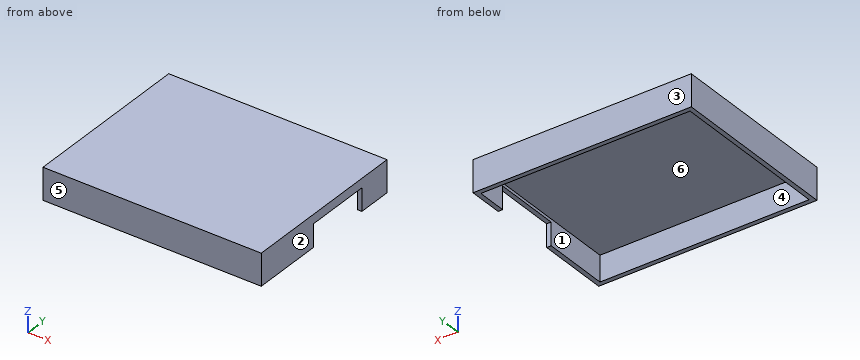
Autodesk Inventor part; units mm, degrees
ref_plane "Plan de construction1" through (-50.5759, 25.8928, -3.5) normal (-1, 0, 0) x (0, 0, 1)
ref_plane "YZ Plane" through (0, 0, 0) normal (1, 0, 0) x (0, 1, 0)
ref_plane "XZ Plane" through (0, 0, 0) normal (0, 1, 0) x (-1, 0, 0)
sketch "Esquisse1" plane through (0, 0, 0) normal (0, 0, 1) x (1, 0, 0)
  line L0 (-45.5759, 93.3928) -> (-189.5759, 93.3928)
  line L1 (-189.5759, 93.3928) -> (-189.5759, -20.6072)
  line L2 (-45.5759, -20.6072) -> (-45.5759, 93.3928)
  line L3 (-189.5759, -20.6072) -> (-45.5759, -20.6072)
  line L4 (-189.5759, 93.3928) -> (-45.5759, 93.3928)
  line L5 (-45.5759, 93.3928) -> (-45.5759, -20.6072)
  line L6 (-45.5759, -20.6072) -> (-189.5759, -20.6072)
  line L7 (-189.5759, -20.6072) -> (-189.5759, 93.3928)
  point P0 (0, 0)
extrude "Extrusion1" add sketch "Esquisse1" along normal blind 21
sketch "Esquisse2" plane through (0, 0, 0) normal (0, 0, -1) x (-1, 0, 0)
  line L0 (186.5759, -17.6072) -> (48.5759, -17.6072)
  line L1 (48.5759, -17.6072) -> (48.5759, 90.3928)
  line L2 (48.5759, 90.3928) -> (186.5759, 90.3928)
  line L3 (186.5759, 90.3928) -> (186.5759, -17.6072)
  line L4 (189.5759, -20.6072) -> (45.5759, -20.6072)
  line L5 (45.5759, 93.3928) -> (189.5759, 93.3928)
  line L6 (189.5759, 93.3928) -> (189.5759, -20.6072)
  line L7 (45.5759, -20.6072) -> (45.5759, 93.3928)
  point P0 (0, 0)
  dimension "d2" = 3
  dimension "d4" = 3
  dimension "d5" = 3
  dimension "d6" = 3
extrude "Extrusion3" cut sketch "Esquisse2" against normal blind 17 contours L0 L1 L2 L3
sketch "Esquisse3" plane through (-45.5759, -20.6072, 0) normal (1, 0, 0) x (0, 0, -1)
  line L0 (-15, 47.25) -> (0, 47.25)
  line L1 (0, 47.25) -> (0, 91.25)
  line L2 (0, 91.25) -> (-15, 91.25)
  line L3 (-15, 91.25) -> (-15, 47.25)
  line L4 (0, -22.8) -> (0, 136.8)
  line L5 (0, 0) -> (-21, 0)
  point P0 (0, 20.6072)
  point P1 (-10.5, -7.9486)
  point P2 (-10.5, 0)
  dimension "d11" = 15
  dimension "d12" = 44
  dimension "d19" = 47.25
ref_plane "Plan de construction1" through (-50.5759, 25.8928, -3.5) normal (-1, 0, 0) x (0, 0, 1)
extrude "Extrusion4" cut sketch "Esquisse3" against normal up to surface (5 mm away)
equation "\"d4\" = d2"
equation "\"d5\" = d2"
equation "\"d6\" = d4"
properties part number "couvercle"
Build history of the part. All positions in model axes, mm. Face numbers are marked on the shaded views. A direction names the side the tool comes from. Round coordinates to 2 decimals unless told otherwise and drop trailing zeros. Write each loop counter-clockwise with the first axis right and the second up, starting at its lowest first coordinate (ties: lowest second). Pieces come first, ordered by that corner, then holes.
1) Band-saw the part on C-C, the plane z = 6.25. List the corners of the cut face in (x, y).
2) Mould opens along X. For the marked faces 1, 2, 3 and 4 say: +X half, -X half, draft (parallel to the pull), parting line (faces both ways), or undercut.
3) Band-saw the part on A-A, the plane y = 30. List the corners of the cut face in (x, z).
4) Pin check, flat tips, straight feed: pin 1 (8.5 mm diameter, centred on y = 34, z = 6, fed in from +X); pin 2 (3 mm diameter, centred on x = -170.5, y = 57.5, fed in from -Z); pin 3 (0.9 mm diameter, centred on x = -47.5, y = 43, fed in from -Z). Stop position of each tip, or through.
5) Band-saw the part on B-B, the plane x = -138.5. List the corners of the cut face in (y, z), and give its area (3 significant figures).
6) 3-axis set-ups, long thin cutter, end or side, ignore diameter. For the marked faces 5 and 6: which of +Z, -Z, +X, -X, +Y, -Y reach the whole face in a straight line?
7) Drill centre lines: probe 1 along Y at (x, z) = (-86, 12.5); probe 2 along X at (y, z) = (-1, 14.25); probe 3 along Z at (x, y) = (-78, 29). Where is each one in solid material? Low to high.
Ans:
1. outline: (-189.58, -20.61) - (-45.58, -20.61) - (-45.58, 26.64) - (-48.58, 26.64) - (-48.58, -17.61) - (-186.58, -17.61) - (-186.58, 90.39) - (-48.58, 90.39) - (-48.58, 70.64) - (-45.58, 70.64) - (-45.58, 93.39) - (-189.58, 93.39) - close
2. face 1: undercut
2. face 2: +X half
2. face 3: draft
2. face 4: undercut
3. outline: (-189.58, 0) - (-186.58, 0) - (-186.58, 17) - (-48.58, 17) - (-48.58, 15) - (-45.58, 15) - (-45.58, 21) - (-189.58, 21) - close
4. pin 1: stops at x = -186.58
4. pin 2: stops at z = 17
4. pin 3: stops at z = 15
5. outline: (-20.61, 0) - (-17.61, 0) - (-17.61, 17) - (90.39, 17) - (90.39, 0) - (93.39, 0) - (93.39, 21) - (-20.61, 21) - close
5. area: 558 mm2
6. face 5: +Z, -Z, +X, -X, -Y
6. face 6: -Z
7. probe 1: y = -20.61 to -17.61, 90.39 to 93.39
7. probe 2: x = -189.58 to -186.58, -48.58 to -45.58
7. probe 3: z = 17 to 21
